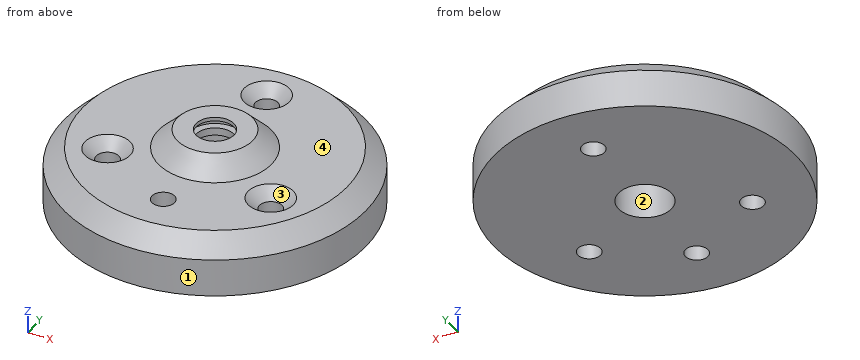
```python
from build123d import *

# Parameters (mm, degrees)
F0_R           = 40
F1_DEPTH       = 15
F2_SIZE        = 5
F3_R           = 15
F4_DEPTH       = 5
F5_SIZE        = 4.99999
F7_D           = 6
F7_CSINK_D     = 12
F7_CSINK_ANGLE = 90
F8_D           = 10.1
F11_D          = 6


# Not quite as in the source:
# - a fillet or chamfer is up to 0.001 mm smaller than in the source, because OpenCascade refuses the exact size


with BuildPart() as f1:
    # F0 (on Top) → F1 (new body)
    with BuildSketch(Plane.XY):
        Circle(F0_R)
    extrude(amount=F1_DEPTH)

    # F2
    f2_edges = [f1.edges().sort_by_distance(p)[0] for p in [
        (-40, 0, 15),
    ]]
    chamfer(f2_edges, length=F2_SIZE)

    # F3 (on face) → F4 (join)
    with BuildSketch(Plane.XY.offset(15)):
        Circle(F3_R)
    extrude(amount=F4_DEPTH)

    # F5 (size 5 in the source; OpenCascade refuses exactly that, so slightly less here)
    f5_edges = [f1.edges().sort_by_distance(p)[0] for p in [
        (-15, 0, 20),
    ]]
    chamfer(f5_edges, length=F5_SIZE)

    # F7 (through all)
    with Locations(Plane.XY.offset(15)):
        with Locations((0, 25), (-21.6506350946, -12.5), (21.6506350946, -12.5)):
            CounterSinkHole(F7_D / 2, F7_CSINK_D / 2, counter_sink_angle=F7_CSINK_ANGLE)

    # F8 (through all)
    with Locations(Plane(origin=(0, 0, 0), x_dir=(1, 0, 0), z_dir=(0, 0, -1))):
        with Locations((0, 0)):
            Hole(F8_D / 2)

    # F9 (on Right) → F10 (revolve, cut)
    with BuildSketch(Plane.YZ):
        Polygon((7, 19), (0, 19), (0, 0), (7, 0), (7, 15), (5.1, 15), (5.1, 17), (7, 17), align=None)
    revolve(axis=Axis((0, 0, 9.5), (0, 0, 1)), mode=Mode.SUBTRACT)

    # F11 (through all)
    with Locations(Plane.XY.offset(15)):
        with Locations((0, -25)):
            Hole(F11_D / 2)


solid = f1.part
```
Verification items for the finished model (mm, model axes). Face numbers are marked on the shaded views. Coordinates: 2 decimals unless noted, no trailing zeros. Loops run counter-clockwise (first coordinate to the right, second up) from the corner with the lowest first, then second, coordinate; pieces in that order, holes last. Notation, with made-up numbers: (-8, 28.5) -> (16, 28.5) arc R20 ccw to (16, 32.5) -> close; hole circle Ø2 at (51.25, 67.5). An arc over 180 degrees is marked (long way). Put each result on its own line as item: value.
1. Mould release check, pull along Y, two halves, no side actions. Record for the marked faces 1, 2, 3 and 4: pulls with the +Y half, pulls with the -Y half, needs draft (parallel to the pull), parting line crosses it, or undercut.
Result set:
face 1: parting line crosses it
face 2: undercut
face 3: undercut
face 4: needs draft
2. Section check C-C, the plane x = 0. Give the number of separate pieces and of enclosed holes in the cut face, then the cut area to 4 significant figures.
Result set:
separate pieces: 4
enclosed holes: 0
area: 842.5 mm^2
3. Gauge pin test, flat ends, axial feed: P1, Ø21, axis at x = 17, y = -17, coming from the +Z side; P2, Ø8, axis at x = 15.5, z = 5, coming from the -Y side; P3, Ø2, axis at x = -8, z = 4, coming from the -Y side. Record the tip position at first contact, or that the pin passes through.
Result set:
P1: stops at z = 16.46
P2: stops at y = -38.31
P3: stops at y = -39.38
4. Thickness scan on line 1 (Y direction, x = 0, z = 6.25); line 2 (X direction, y = -12.5, z = 6.5); line 3 (Z direction, x = -24.5, y = 16). Record the ranges inside material, lowest first.
Result set:
line 1: y = -40 to -28, -22 to -7, 7 to 22, 28 to 40
line 2: x = -38 to -24.65, -18.65 to 18.65, 24.65 to 38
line 3: z = 0 to 15
5. Section check B-B, the plane z = 2.5. Record the boundary of the cut face in (x, y), then the cut area to 3 significant figures.
Result set:
outline: circle Ø80 at (0, 0); hole circle Ø6 at (-21.65, -12.5); hole circle Ø14 at (0, 0); hole circle Ø6 at (0, -25); hole circle Ø6 at (0, 25); hole circle Ø6 at (21.65, -12.5)
area: 4,760 mm^2
